from build123d import *

# Parameters (mm, degrees)
LINEAR_AUSTRAGEN_D_NN1_DEPTH    = 5
VERRUNDUNG1_R                   = 5
VERRUNDUNG2_R                   = 1
VERRUNDUNG3_R                   = 0.1
SKIZZE2_R                       = 2.5
SCHNITT_LINEAR_AUSTRAGEN1_DEPTH = 10
SCHNITT_LINEAR_AUSTRAGEN2_DEPTH = 10


with BuildPart() as part:
    # Skizze1 → Linear-Austragen-Dünn1 (new, symmetric)
    with BuildSketch(Plane.XY):
        Polygon((0, 15), (0, 0), (-15, 0), (-15, -1), (1, -1), (1, 15), align=None)
    extrude(amount=LINEAR_AUSTRAGEN_D_NN1_DEPTH, both=True)

    # Verrundung1
    verrundung1_edges = [part.edges().sort_by_distance(p)[0] for p in [
        (-15, -0.5, -5),
        (-15, -0.5, 5),
        (0.5, 15, -5),
        (0.5, 15, 5),
    ]]
    fillet(verrundung1_edges, radius=VERRUNDUNG1_R - 0.0001)  # a hair under: the kernel refuses the full size

    # Verrundung2
    verrundung2_edges = [part.edges().sort_by_distance(p)[0] for p in [
        (1, -1, 0),
    ]]
    fillet(verrundung2_edges, radius=VERRUNDUNG2_R)

    # Verrundung3
    verrundung3_edges = [part.edges().sort_by_distance(p)[0] for p in [
        (0, 0, 0),
    ]]
    fillet(verrundung3_edges, radius=VERRUNDUNG3_R)

    # Skizze2 → Schnitt-Linear austragen1 (cut)
    with BuildSketch(Plane.ZY):
        with Locations(Location((0, 10, 0), (0, 0, 270))):
            Circle(SKIZZE2_R)
    extrude(amount=-SCHNITT_LINEAR_AUSTRAGEN1_DEPTH, mode=Mode.SUBTRACT)

    # Skizze3 → Schnitt-Linear austragen2 (cut)
    with BuildSketch(Plane(origin=(0, 0, 0), x_dir=(1, 0, 0), z_dir=(0, 1, 0))):
        with BuildLine():
            Line((-10, 2.5), (-5, 2.5))
            ThreePointArc((-5, 2.5), (-2.5, 0), (-5, -2.5))
            Line((-5, -2.5), (-10, -2.5))
            ThreePointArc((-10, -2.5), (-12.5, 0), (-10, 2.5))
        make_face()
    extrude(amount=-SCHNITT_LINEAR_AUSTRAGEN2_DEPTH, mode=Mode.SUBTRACT)


solid = part.part
Design review of the part built by this model. Coordinates are the model's own, in mm. A direction names the side the tool comes from. Coordinates: 2 decimals unless noted, no trailing zeros. Order: outer loops, then holes, each group sorted by start corner. A loop starts at its lowest first (then second) coordinate and runs counter-clockwise, first axis right, second up.
Item 1: For line 1 (Z direction, x = 0.6, y = 10); line 2 (Y direction, x = -11, z = 4.5); line 3 (X direction, y = 2, z = -1), list the stretches that pass through material, from the lowest coordinate up.
Item 2: Take a section at B-B, the plane y = 11. Write out the cut boundary in (x, z), then the cut area to 3 significant figures.
Item 3: The part is to be moulded in two halves that separate along Y. For faces 4 (the cylindrical face through (0.5, 12.5, 0.1)), 5 (the cylindrical face through (-13.57, -0.51, 3.5)), 6 (the flat face through (-8, -1, -3)), 7 (the flat face through (-7, 0, -3)), say which applies: pulls with the +Y half, pulls with the -Y half, needs draft (parallel to the pull), parting line crosses it, or undercut.
Item 4: Take a section at C-C, the plane z = 1.5. Write out the cut boundary in (x, y), then the cut area to 3 significant figures.
Item 5: Take a section at D-D, the plane z = 4. Write out the cut boundary in (x, y).
Item 6: For pin 1 Ø6 at (y, z) = (4.5, 3) entering from -X; pin 2 Ø5 at (x, z) = (-7, -2) entering from +Y, all flat-tipped, find the tip position at first contact; note any pin that passes through.
Item 7: For faces 1 (the flat face through (0, 6, 0)), 2 (the flat face through (-7.5, -0.5, 2.5)), 3 (the cylindrical face through (0.49, 13.57, 3.5)), list the 3-axis set-ups (+Z, -Z, +X, -X, +Y, -Y) from which the entire face can be reached by the end or side of a thin tool; tool diameter is ignored.
Item 8: Take a section at A-A, the plane x = -8.5. Write out the cut boundary in (y, z), then the cut area to 3 significant figures.
The answers:
1. line 1: z = -5 to -2.5, 2.5 to 5
1. line 2: y = -1 to 0
1. line 3: x = 0 to 1
2. outline: (0, -4.9) - (1, -4.9) - (1, -2.29) - (0, -2.29) - close; (0, 2.29) - (1, 2.29) - (1, 4.9) - (0, 4.9) - close
2. area: 5.22 mm2
3. face 4: undercut
3. face 5: needs draft
3. face 6: pulls with the -Y half
3. face 7: pulls with the +Y half
4. outline: (-14.77, -1) - (-12, -1) - (-12, 0) - (-14.77, 0) - close; (-3, -1) - (0, -1) arc R1 ccw to (1, 0) - (1, 8) - (0, 8) - (0, 0.1) arc R0.1 cw to (-0.1, 0) - (-3, 0) - close; (0, 12) - (1, 12) - (1, 14.77) - (0, 14.77) - close
4. area: 17.3 mm2
5. outline: (-13, -1) - (0, -1) arc R1 ccw to (1, 0) - (1, 13) - (0, 13) - (0, 0.1) arc R0.1 cw to (-0.1, 0) - (-13, 0) - close
6. pin 1: stops at x = 0
6. pin 2: stops at y = 0
7. face 1: +Z, -Z, -X, +Y
7. face 2: +Y, -Y
7. face 3: +Z, +X, -X, +Y
8. outline: (-1, -5) - (0, -5) - (0, -2.5) - (-1, -2.5) - close; (-1, 2.5) - (0, 2.5) - (0, 5) - (-1, 5) - close
8. area: 5.00 mm2
